Read the model definition and answer for the solid it produces. Units are mm, in the model's axes. A direction names the side the tool comes from. Round coordinates to 2 decimals unless told otherwise and drop trailing zeros. Order: outer loops, then holes, each group sorted by start corner. A loop starts at its lowest first (then second) coordinate and runs counter-clockwise, first axis right, second up. Notation, with made-up numbers: (8.25, 7.5) -> (50.25, 7.5) arc R16 cw to (50.25, 14.5) -> close; hole circle Ø4 at (53, 26.5). An arc over 180 degrees is marked (long way). One line per item, written item: value. Start each with the question number.
1. For faces 1 (the face through (-25, 14, -6.35)), 2 (the face through (24, 8.5, -5)), 3 (the face through (0, 14, 10.2)), determine the directions among +Z, -Z, +X, -X, +Y, -Y from which every point of the face is accessible in a straight line to the end or side of a thin tool.
2. The mould has two halves that part along X. Classify faces 4 (the face through (-30, 14, 13)), 5 (the face through (30, 14, 0)), 6 (the face through (26.474, 14.05, 13.648)), 7 (the face through (7, 0, -13)): released by +X, released by -X, zero draft, split by the parting line, or undercut.
3. Section C-C (z = 15) is taken. Give the vertices of the cut face in (x, y).
4. Flat-ended cylindrical pins translate along their axes: pin 1 Ø6 at (y, z) = (10.5, -1.5) entering from -X; pin 2 Ø1.5 at (x, z) = (24, -5) entering from +Y. Find the tip coordinate at first contact, or state that the pin passes through.
5. Section A-A (x = -17) is taken. Give the vertices of the cut face in (y, z).
6. Section B-B (y = 14.25) is taken. Give the vertices of the cut face in (x, z).
7. Consider line 1 (Z direction, x = -25, y = 14.5); line 2 (Z direction, x = 24.25, y = 24.25); line 3 (Z direction, x = -12.5, y = 21.75). Determine where each line is inside the solid, lowest interval first.
8. Section D-D (y = 3.75) is taken. Give the vertices of the cut face in (x, z).
Autodesk Inventor part; units mm, degrees
ref_plane "YZ Plane" through (0, 0, 0) normal (1, 0, 0) x (0, 1, 0)
ref_plane "XZ Plane" through (0, 0, 0) normal (0, 1, 0) x (-1, 0, 0)
ref_plane "XY Plane" through (0, 0, 0) normal (0, 0, 1) x (1, 0, 0)
sketch "Sketch1" plane through (0, 0, 0) normal (0, 1, 0) x (-1, 0, 0)
  line L0 (-20.2, -10.2) -> (20.2, -10.2)
  line L1 (20.2, -10.2) -> (20.2, 10.2)
  line L2 (20.2, 10.2) -> (-20.2, 10.2)
  line L3 (-20.2, 10.2) -> (-20.2, -10.2)
  line L4 (-20.2, -10.2) -> (20.2, 10.2) construction
  line L5 (20.2, -10.2) -> (-20.2, 10.2) construction
  line L6 (-30, -20) -> (30, -20)
  line L7 (30, -20) -> (30, 20)
  line L8 (30, 20) -> (-30, 20)
  line L9 (-30, 20) -> (-30, -20)
  line L10 (-30, -20) -> (30, 20) construction
  line L11 (30, -20) -> (-30, 20) construction
  circle A0 centre (25, 15) radius 2
  circle A1 centre (25, -15) radius 2
  circle A2 centre (-25, 15) radius 2
  circle A3 centre (-25, -15) radius 2
  point P0 (0, 0)
  dimension "d0" = 20.4
  dimension "d1" = 40.4
  dimension "d2" = 60
  dimension "d3" = 40
  dimension "d4" = 4
  dimension "d5" = 4
  dimension "d7" = 4
  dimension "d8" = 5
  dimension "d9" = 5
  dimension "d10" = 5
  dimension "d11" = 5
  dimension "d13" = 4
  dimension "d14" = 5
  dimension "d15" = 5
  dimension "d16" = 5
  dimension "d17" = 5
extrude "Extrusion1" add sketch "Sketch1" along normal blind 28.5
sketch "Sketch2" plane through (0, 28.5, 0) normal (0, 1, 0) x (1, 0, 0)
  circle A0 centre (-24.25, -4.75) radius 1.5
  circle A1 centre (-24.25, 4.75) radius 1.5
  circle A2 centre (24.25, -4.75) radius 1.5
  circle A3 centre (24.25, 4.75) radius 1.5
  line L0 (20.2, 10.2) -> (20.2, -10.2)
  point P0 (0, 0)
  point P1 (20.2, 0)
  dimension "d20" = 3
  dimension "d21" = 3
  dimension "d22" = 3
  dimension "d23" = 3
  dimension "d24" = 48.5
  dimension "d25" = 24.25
  dimension "d26" = 48.5
  dimension "d27" = 24.25
  dimension "d28" = 9.5
  dimension "d29" = 4.75
  dimension "d30" = 9.5
  dimension "d31" = 4.75
extrude "Extrusion2" cut sketch "Sketch2" against normal blind 20
sketch "Sketch3" plane through (0, 28.5, 0) normal (0, 1, 0) x (1, 0, 0)
  line L0 (-30, 20) -> (-30, -20)
  line L1 (-20.2, -10.2) -> (-20.2, 10.2)
  line L2 (-30, 6.3495) -> (-20.2, 6.3495)
  line L3 (-20.2, 6.3495) -> (-20.2, -6.2601)
  line L4 (-20.2, -6.2601) -> (-30, -6.2601)
  line L5 (-30, -6.2601) -> (-30, 6.3495)
  point P0 (0, 0)
  point P1 (-20.2, 6.3495)
extrude "Extrusion3" cut sketch "Sketch3" against normal through all
properties part number "Servoholder"
Answer:
1. face 1: -X, +Y, -Y
1. face 2: +Y
1. face 3: +Y, -Y
2. face 4: released by -X
2. face 5: released by +X
2. face 6: undercut
2. face 7: zero draft
3. outline: (-30, 0) -> (-27, 0) -> (-27, 28.5) -> (-30, 28.5) -> close; (-23, 0) -> (23, 0) -> (23, 28.5) -> (-23, 28.5) -> close; (27, 0) -> (30, 0) -> (30, 28.5) -> (27, 28.5) -> close
4. pin 1: x = 20.2
4. pin 2: y = 8.5
5. outline: (0, -20) -> (28.5, -20) -> (28.5, -10.2) -> (0, -10.2) -> close; (0, 10.2) -> (28.5, 10.2) -> (28.5, 20) -> (0, 20) -> close
6. outline: (-30, -20) -> (30, -20) -> (30, 20) -> (-30, 20) -> (-30, 6.26) -> (-20.2, 6.26) -> (-20.2, 10.2) -> (20.2, 10.2) -> (20.2, -10.2) -> (-20.2, -10.2) -> (-20.2, -6.35) -> (-30, -6.35) -> close; hole circle Ø4 at (-25, -15); hole circle Ø4 at (-25, 15); hole circle Ø3 at (24.25, -4.75); hole circle Ø3 at (24.25, 4.75); hole circle Ø4 at (25, -15); hole circle Ø4 at (25, 15)
7. line 1: -20 to -17, -13 to -6.35, 6.26 to 13, 17 to 20
7. line 2: -20 to -16.85, -13.15 to -6.25, -3.25 to 3.25, 6.25 to 13.15, 16.85 to 20
7. line 3: -20 to -10.2, 10.2 to 20
8. outline: (-30, -20) -> (30, -20) -> (30, 20) -> (-30, 20) -> (-30, 6.26) -> (-20.2, 6.26) -> (-20.2, 10.2) -> (20.2, 10.2) -> (20.2, -10.2) -> (-20.2, -10.2) -> (-20.2, -6.35) -> (-30, -6.35) -> close; hole circle Ø4 at (-25, -15); hole circle Ø4 at (-25, 15); hole circle Ø4 at (25, -15); hole circle Ø4 at (25, 15)
